For this review, take the finished solid that the model builds, in its own axes (mm). Face numbers are marked on the shaded views. A direction names the side the tool comes from. Coordinates: 2 decimals unless noted, no trailing zeros. Write each loop counter-clockwise with the first axis right and the second up, starting at its lowest first coordinate (ties: lowest second). Pieces come first, ordered by that corner, then holes. Notation, with made-up numbers: (65, 78) - (70, 78) arc R27 ccw to (70, 105) - close; hole circle Ø6 at (-11, 43). An arc over 180 degrees is marked (long way). Use one line per item in the form item = value. Start each with the question number.
1) We need section A-A (y = 3.5). Give the boundary of the cut face in (x, z), plus the area to 3 significant figures.
2) We need section C-C (y = 26.5). Give the boundary of the cut face in (x, z), plus the area to 3 significant figures.
3) Insertion check: P1, Ø13, axis at x = 0, y = 36, coming from the -Z side; P2, Ø1.6, axis at x = 10, z = -27, coming from the +Y side; P3, Ø3.5, axis at x = -22, z = -106, coming from the +Y side. Each pin has a flat end and moves straight along its axis. Give the tip position at first contact, or say it passes through.
4) We need section D-D (x = 5). Give the boundary of the cut face in (y, z) (3 decimals).
5) For L1, parallel to Z at x = -22, y = 2.5; L2, parallel to X at y = 4, z = -36; L3, parallel to Y at x = 0, z = -126, list the stretches that pass through material, from the lowest coordinate up. Write a range as from..to.
6) We need section B-B (z = -49). Give the boundary of the cut face in (x, y).
7) Tool access review of the marked faces 4, 5, 6, 7 and 8: name each direction out of +Z, -Z, +X, -X, +Y, -Y from which nothing blocks a thin tool from reaching the whole face with its end or side.
8) Mouldability with a two-part tool opening along Y and no side actions: class the marked faces 1, 2 and 3 as pulls with the +Y half, pulls with the -Y half, needs draft (parallel to the pull), parting line crosses it, or undercut.
```python
from build123d import *

# Parameters (mm, degrees)
BOSS_EXTRUDE1_DEPTH = 32
SKETCH2_R           = 3
CUT_EXTRUDE1_DEPTH  = 10
CHAMFER2_SIZE       = 3
CHAMFER3_SIZE       = 3
CHAMFER4_SIZE       = 3
CHAMFER5_SIZE       = 3
CUT_EXTRUDE3_DEPTH  = 145
CUT_EXTRUDE4_REACH  = 146
SKETCH7_R           = 8
CUT_EXTRUDE8_REACH  = 146
FILLET1_R           = 3
SKETCH9_W           = 64
SKETCH9_H           = 4
BOSS_EXTRUDE2_DEPTH = 2


with BuildPart() as part:
    # Sketch1 → Boss-Extrude1 (new body, symmetric)
    with BuildSketch(Plane(origin=(0, 0, 0), x_dir=(0, 0, -1), z_dir=(1, 0, 0))):
        Polygon((0, 0), (0, 36), (16, 52), (26, 52), (26, 16), (122, 16), (122, 52), (144, 52), (144, 0), align=None)
    extrude(amount=BOSS_EXTRUDE1_DEPTH, both=True)

    # Sketch2 → Cut-Extrude1 (cut)
    with BuildSketch(Plane(origin=(0, 0, 0), x_dir=(1, 0, 0), z_dir=(0, 1, 0))):
        with Locations((-22, 36)):
            Circle(SKETCH2_R)
        with Locations((22, 36)):
            Circle(SKETCH2_R)
        with Locations((-22, 106)):
            Circle(SKETCH2_R)
        with Locations((22, 106)):
            Circle(SKETCH2_R)
    extrude(amount=CUT_EXTRUDE1_DEPTH, mode=Mode.SUBTRACT)

    # Chamfer2
    chamfer2_edges = [part.edges().sort_by_distance(p)[0] for p in [
        (19, 10, -106),
    ]]
    chamfer(chamfer2_edges, length=CHAMFER2_SIZE)

    # Chamfer3
    chamfer3_edges = [part.edges().sort_by_distance(p)[0] for p in [
        (-25, 10, -106),
    ]]
    chamfer(chamfer3_edges, length=CHAMFER3_SIZE)

    # Chamfer4
    chamfer4_edges = [part.edges().sort_by_distance(p)[0] for p in [
        (19, 10, -36),
    ]]
    chamfer(chamfer4_edges, length=CHAMFER4_SIZE)

    # Chamfer5
    chamfer5_edges = [part.edges().sort_by_distance(p)[0] for p in [
        (-25, 10, -36),
    ]]
    chamfer(chamfer5_edges, length=CHAMFER5_SIZE)

    # Sketch6 → Cut-Extrude3 (cut, through all)
    with BuildSketch(Plane.XY):
        Polygon((-16, 0), (-16, 7), (-8, 7), (-8, 16), (0, 16), (8, 16), (8, 7), (16, 7), (16, 0), align=None)
    extrude(amount=-CUT_EXTRUDE3_DEPTH, mode=Mode.SUBTRACT)

    # Sketch7 → Cut-Extrude4 (cut, up to next)
    with BuildSketch(Plane(origin=(0, 0, -144), x_dir=(-1, 0, 0), z_dir=(0, 0, -1)), mode=Mode.PRIVATE) as cut_extrude4_sk1:
        with Locations((0, 36)):
            Circle(SKETCH7_R)
    cut_extrude4_tool1 = extrude(cut_extrude4_sk1.sketch, amount=-CUT_EXTRUDE4_REACH, mode=Mode.PRIVATE) & part.part
    add(cut_extrude4_tool1.solids().sort_by_distance((0, 36, -144))[0], mode=Mode.SUBTRACT)

    # Sketch8 → Cut-Extrude8 (cut, up to next)
    with BuildSketch(Plane(origin=(0, 0, -144), x_dir=(-1, 0, 0), z_dir=(0, 0, -1)), mode=Mode.PRIVATE) as cut_extrude8_sk1:
        with BuildLine():
            Line((-32, 16), (-27.596884244, 16))
            Line((-27.596884244, 16), (-14.372185951, 43.031377602))
            ThreePointArc((-14.372185951, 43.031377602), (-8.470476894, 49.573909576), (5.2e-08, 52))
            Line((5.2e-08, 52), (-32, 52))
            Line((-32, 52), (-32, 16))
        make_face()
    cut_extrude8_tool1 = extrude(cut_extrude8_sk1.sketch, amount=-CUT_EXTRUDE8_REACH, mode=Mode.PRIVATE) & part.part
    add(cut_extrude8_tool1.solids().sort_by_distance((23.880103, 38.416138, -144))[0], mode=Mode.SUBTRACT)
    # Sketch8 → Cut-Extrude8 (cut, up to next)
    with BuildSketch(Plane(origin=(0, 0, -144), x_dir=(-1, 0, 0), z_dir=(0, 0, -1)), mode=Mode.PRIVATE) as cut_extrude8_sk2:
        with BuildLine():
            Line((14.372185951, 43.031377602), (27.596884244, 16))
            Line((27.596884244, 16), (32, 16))
            Line((32, 16), (32, 52))
            Line((32, 52), (5.2e-08, 52))
            ThreePointArc((5.2e-08, 52), (8.470476938, 49.573909549), (14.372185951, 43.031377602))
        make_face()
    cut_extrude8_tool2 = extrude(cut_extrude8_sk2.sketch, amount=-CUT_EXTRUDE8_REACH, mode=Mode.PRIVATE) & part.part
    add(cut_extrude8_tool2.solids().sort_by_distance((-23.880103, 38.416138, -144))[0], mode=Mode.SUBTRACT)

    # Fillet1
    fillet1_edges = [part.edges().sort_by_distance(p)[0] for p in [
        (-27.596884244, 16, -133),
        (27.596884244, 16, -133),
    ]]
    fillet(fillet1_edges, radius=FILLET1_R)

    # Sketch9 → Boss-Extrude2 (add)
    with BuildSketch(Plane(origin=(0, 0, -26), x_dir=(-1, 0, 0), z_dir=(0, 0, -1))):
        with Locations((0, 46)):
            Rectangle(SKETCH9_W, SKETCH9_H)
    extrude(amount=BOSS_EXTRUDE2_DEPTH)


solid = part.part
```
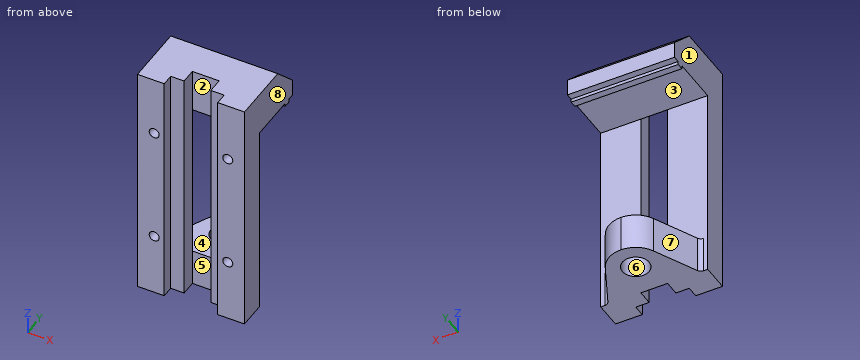
Determined:
q1.outline = (-32, -144) - (-16, -144) - (-16, 0) - (-32, 0) - close; (16, -144) - (32, -144) - (32, 0) - (16, 0) - close; hole circle Ø6 at (-22, -106); hole circle Ø6 at (-22, -36); hole circle Ø6 at (22, -106); hole circle Ø6 at (22, -36)
q1.area = 4,490 mm²
q2.outline = (-32, -26) - (32, -26) - (32, 0) - (-32, 0) - close; (-22.46, -144) - (22.46, -144) - (22.46, -122) - (-22.46, -122) - close
q2.area = 2,650 mm²
q3.P1 = -26
q3.P2 = 48
q3.P3 = 16
q4.outline = (16, -144) - (29.755, -144) - (29.755, -122) - (16, -122) - close; (16, -26) - (44, -26) - (44, -28) - (48, -28) - (48, -26) - (52, -26) - (52, -16) - (36, 0) - (16, 0) - close; (42.245, -144) - (51.199, -144) - (51.199, -122) - (42.245, -122) - close
q5.L1 = -144..-109, -103..-39, -33..0
q5.L2 = -32..-25, -19..-16, 16..19, 25..32
q5.L3 = 16..28, 44..52
q6.outline = (-32, 0) - (-16, 0) - (-16, 7) - (-8, 7) - (-8, 16) - (-32, 16) - close; (8, 7) - (16, 7) - (16, 0) - (32, 0) - (32, 16) - (8, 16) - close
q7.face_4 = +X, -X, +Y
q7.face_5 = +Z, -Z, -Y
q7.face_6 = -Z
q7.face_7 = -Z, -X, +Y
q7.face_8 = +Z, -Z, +X, +Y, -Y
q8.face_1 = needs draft
q8.face_2 = pulls with the -Y half
q8.face_3 = undercut
